```python
from build123d import *

# Parameters (mm, degrees)
EXTRUDE_START       = -10
SKETCH_3_W          = 150
SKETCH_3_H          = 80
EXTRUDE_3_DEPTH     = 10
SKETCH_5_R          = 2.5
EXTRUDE_5_DEPTH     = 22.5
SKETCH_6_W          = 53.56449621
SKETCH_6_H          = 15
SKETCH_6_W_2        = 55.316324433
SKETCH_6_H_2        = 5
SKETCH_6_W_3        = 50.048103058
CUT_EXTRUDE_1_DEPTH = 40
SKETCH_7_R          = 2.5
EXTRUDE_6_DEPTH     = 17.5
SKETCH_4_R          = 2.5
EXTRUDE_4_DEPTH     = 7.5
EXTRUDE_START_2     = -17.5
SKETCH_9_R          = 2.5
EXTRUDE_7_DEPTH     = 15
SKETCH_8_W          = 149.834413798
SKETCH_8_H          = 5
SKETCH_8_W_2        = 53.466456482
SKETCH_8_W_3        = 46.484368984
SKETCH_8_W_4        = 21.970588524
CUT_EXTRUDE_2_DEPTH = 35


with BuildPart() as part:
    # 草圖3 → 填料-伸長3 (new body)
    with BuildSketch(Plane(origin=(0, 0, 0), x_dir=(1, 0, 0), z_dir=(0, 1, 0)).offset(EXTRUDE_START)):
        with Locations((33.25, 0)):
            Rectangle(SKETCH_3_W, SKETCH_3_H)
    extrude(amount=-EXTRUDE_3_DEPTH)

    # 草圖5 → 填料-伸長5 (add, symmetric)
    with BuildSketch(Plane.XY):
        with BuildLine():
            Line((-11.366060556, 1.149545417), (-14, -10))
            Line((-14, -10), (1, -10))
            Line((1, -10), (-1.633939444, 1.149545417))
            ThreePointArc((-1.633939444, 1.149545417), (-6.5, 5), (-11.366060556, 1.149545417))
        make_face()
        with Locations((-6.5, 0)):
            Circle(SKETCH_5_R, mode=Mode.SUBTRACT)
    extrude(amount=EXTRUDE_5_DEPTH, both=True)

    # 草圖6 → 除料-伸長1 (cut)
    with BuildSketch(Plane(origin=(0, -10, 0), x_dir=(1, 0, 0), z_dir=(0, 1, 0))):
        with Locations((-2.489143795, 0)):
            Rectangle(SKETCH_6_W, SKETCH_6_H)
        with Locations((-4.247340371, -15)):
            Rectangle(SKETCH_6_W_2, SKETCH_6_H_2)
        with Locations((-1.613229684, 15)):
            Rectangle(SKETCH_6_W_3, SKETCH_6_H_2)
    extrude(amount=CUT_EXTRUDE_1_DEPTH, mode=Mode.SUBTRACT)

    # 草圖7 → 填料-伸長6 (add, symmetric)
    with BuildSketch(Plane.XY):
        with BuildLine():
            Line((58.633939444, 1.149545417), (56, -10))
            Line((56, -10), (71, -10))
            Line((71, -10), (68.366060556, 1.149545417))
            ThreePointArc((68.366060556, 1.149545417), (63.5, 5), (58.633939444, 1.149545417))
        make_face()
        with Locations((63.5, 0)):
            Circle(SKETCH_7_R, mode=Mode.SUBTRACT)
        with BuildLine():
            Line((38.517037013, 20.412407413), (36, -10))
            Line((36, -10), (51, -10))
            Line((51, -10), (48.482962987, 20.412407413))
            ThreePointArc((48.482962987, 20.412407413), (43.5, 25), (38.517037013, 20.412407413))
        make_face()
        with Locations((43.5, 20)):
            Circle(SKETCH_7_R, mode=Mode.SUBTRACT)
    extrude(amount=EXTRUDE_6_DEPTH, both=True)

    # 草圖4 → 填料-伸長4 (add, symmetric)
    with BuildSketch(Plane.XY):
        with BuildLine():
            Line((87.176081429, -0.184777731), (84.5, -10))
            Line((84.5, -10), (99.5, -10))
            Line((99.5, -10), (96.823918571, -0.184777731))
            ThreePointArc((96.823918571, -0.184777731), (92, 3.5), (87.176081429, -0.184777731))
        make_face()
        with Locations((92, -1.5)):
            Circle(SKETCH_4_R, mode=Mode.SUBTRACT)
        with BuildLine():
            Line((-20.402832148, 2.980936759), (-23, -10))
            Line((-23, -10), (-8, -10))
            Line((-8, -10), (-10.597167852, 2.980936759))
            ThreePointArc((-10.597167852, 2.980936759), (-15.5, 7), (-20.402832148, 2.980936759))
        make_face()
        with Locations((-15.5, 2)):
            Circle(SKETCH_4_R, mode=Mode.SUBTRACT)
        with BuildLine():
            Line((19.133939444, 1.149545417), (16.5, -10))
            Line((16.5, -10), (31.5, -10))
            Line((31.5, -10), (28.866060556, 1.149545417))
            ThreePointArc((28.866060556, 1.149545417), (24, 5), (19.133939444, 1.149545417))
        make_face()
        with Locations((24, 0)):
            Circle(SKETCH_4_R, mode=Mode.SUBTRACT)
    extrude(amount=EXTRUDE_4_DEPTH, both=True)

    # 草圖9 → 填料-伸長7 (add)
    with BuildSketch(Plane.XY.offset(EXTRUDE_START_2)):
        with BuildLine():
            Line((5.045078047, 11.169886883), (2.182988659, -10))
            Line((2.182988659, -10), (17.817011341, -10))
            Line((17.817011341, -10), (14.954921953, 11.169886883))
            ThreePointArc((14.954921953, 11.169886883), (10, 15.5), (5.045078047, 11.169886883))
        make_face()
        with Locations((10, 10.5)):
            Circle(SKETCH_9_R, mode=Mode.SUBTRACT)
    extrude(amount=-EXTRUDE_7_DEPTH)

    # 草圖8 → 除料-伸長2 (cut)
    with BuildSketch(Plane(origin=(0, -10, 0), x_dir=(1, 0, 0), z_dir=(0, 1, 0))):
        with Locations((38.363273687, 0)):
            Rectangle(SKETCH_8_W, SKETCH_8_H)
        with Locations((60.98088391, 10)):
            Rectangle(SKETCH_8_W_2, SKETCH_8_H)
        with Locations((56.879490972, -10)):
            Rectangle(SKETCH_8_W_3, SKETCH_8_H)
        with Locations((12.54422866, 25)):
            Rectangle(SKETCH_8_W_4, SKETCH_8_H)
    extrude(amount=CUT_EXTRUDE_2_DEPTH, mode=Mode.SUBTRACT)


solid = part.part
```
Model file for the job. Use its own axes, mm. A direction names the side the tool comes from. Give positions to 0.01 mm unless a question says otherwise; leave off trailing zeros. Loops run counter-clockwise (first coordinate to the right, second up) from the corner with the lowest first, then second, coordinate; pieces in that order, holes last. Notation, with made-up numbers: (63, 32) - (73, 32) arc R20 cw to (73, 43) - close; hole circle Ø10 at (79.25, -10.75). An arc over 180 degrees is marked (long way). One line per item, written item: value. Start each with the question number.
1. Pull direction Z, two halves, no side cores. Call faces 4 (the flat face through (-5, -3, 7.5)), 5 (the flat face through (57.335, -4.347, 14.965)), 6 (the flat face through (32, -15, 40)), 7 (the flat face through (43, 3, -2.5)): pulls with the +Z half, pulls with the -Z half, needs draft (parallel to the pull), parting line crosses it, or undercut.
2. Probe L1, parallel to Z at x = 46, y = 14; L2, parallel to Y at x = -6.5, z = -21.3; L3, parallel to X at y = 20, z = 15. List the from-to ranges inside material, lowest first. Write a range as from..to.
3. Slice it at C-C (x = -6.5). Give the number of separate pieces and of enclosed holes in the cut face, plus the area to 3 significant figures.
4. Slice it at A-A (x = 10). List the corners of the cut face in (y, z).
5. Slice it at B-B (z = 10.5). List the corners of the cut face in (x, y), plus the area to 3 significant figures.
6. Which spindle directions (+Z, -Z, +X, -X, +Y, -Y) get a long thin tool onto all of the face, cutting with end or side? Do faces 1 (the flat face through (-7, -4, 12.5)), 2 (the flat face through (-12.665, -4.347, 10.035)), 3 (the flat face through (43, 3, -7.5)). Say none if no direction does.
7. Pin check, flat tips, straight feed: pin 1 (12 mm diameter, centred on x = 60.5, y = -3.5, fed in from +Z); pin 2 (3.5 mm diameter, centred on x = -19, y = 0.5, fed in from +Z); pin 3 (8 mm diameter, centred on y = 20.5, z = 8.5, fed in from -X); pin 4 (3 mm diameter, centred on x = 43.5, y = 20, fed in from -Z). Stop position of each tip, or through.
Solution:
1. face 4: undercut
1. face 5: needs draft
1. face 6: pulls with the +Z half
1. face 7: undercut
2. L1: z = -17.5..-12.5, -7.5..-2.5, 2.5..7.5, 12.5..17.5
2. L2: y = -20..-2.5, 2.5..5
2. L3: x = 38.48..41, 46..48.52
3. separate pieces: 5
3. enclosed holes: 0
3. area: 1,000 mm^2
4. outline: (-20, -40) - (-10, -40) - (-10, -32.5) - (8, -32.5) - (8, -27.5) - (-10, -27.5) - (-10, -22.5) - (8, -22.5) - (8, -17.5) - (-10, -17.5) - (-10, 40) - (-20, 40) - close; (13, -32.5) - (15.5, -32.5) - (15.5, -27.5) - (13, -27.5) - close; (13, -22.5) - (15.5, -22.5) - (15.5, -17.5) - (13, -17.5) - close
5. outline: (-41.75, -20) - (108.25, -20) - (108.25, -10) - (1, -10) - (-1.63, 1.15) arc R5 ccw to (-11.37, 1.15) - (-14, -10) - (-41.75, -10) - close; hole circle Ø5 at (-6.5, 0)
5. area: 1,650 mm^2
6. face 1: -X, +Y
6. face 2: +Z, -X, +Y
6. face 3: +X, +Y
7. pin 1: stops at z = 17.5
7. pin 2: stops at z = 7.5
7. pin 3: stops at x = 38.2
7. pin 4: passes through
